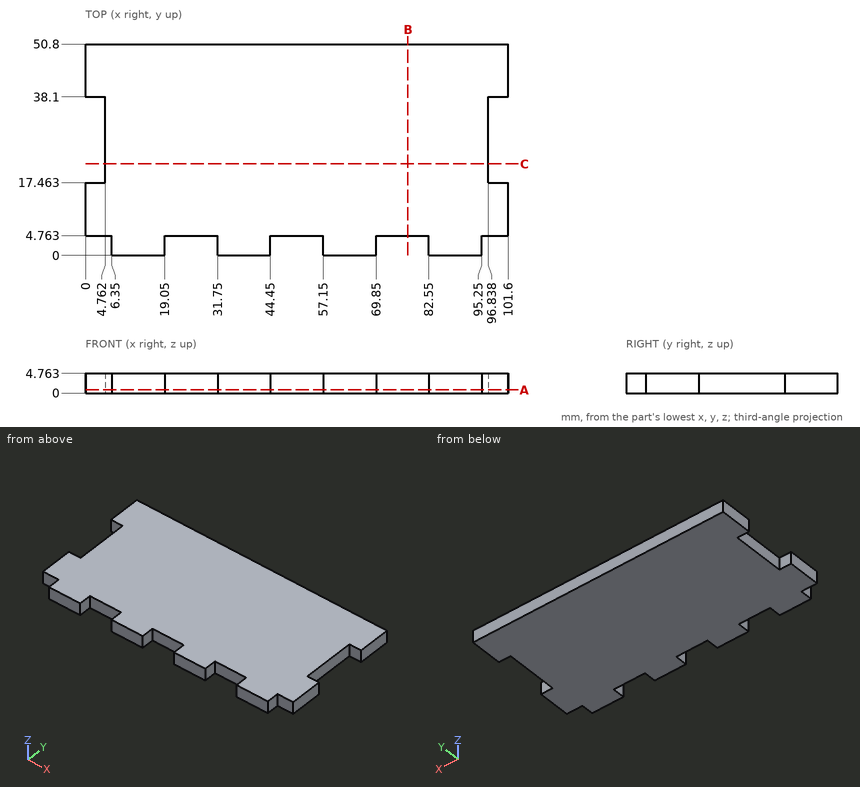
Design review of the part shown in the three views and the two pictorial views. Dimensions are in mm from the part's minimum x, y and z. Round coordinates to 2 decimals unless told otherwise and drop trailing zeros. Write each loop counter-clockwise with the first axis right and the second up, starting at its lowest first coordinate (ties: lowest second). Pieces come first, ordered by that corner, then holes. Notation, with made-up numbers: (28, 54) -> (75, 54) arc R26 cw to (75, 71) -> close; hole circle Ø2 at (19, -11). An arc over 180 degrees is marked (long way). Answer as a JSON object with one key per item and string values.
1. We need section C-C on y = 22. State the section outline as (x, z) points.
Results found:
{"outline": "(4.76, 0) -> (96.84, 0) -> (96.84, 4.76) -> (4.76, 4.76) -> close"}
2. We need section A-A on z = 0.8. State the section outline as (x, y) points, and give its area (3 significant figures).
Results found:
{"outline": "(0, 4.76) -> (6.35, 4.76) -> (6.35, 0) -> (19.05, 0) -> (19.05, 4.76) -> (31.75, 4.76) -> (31.75, 0) -> (44.45, 0) -> (44.45, 4.76) -> (57.15, 4.76) -> (57.15, 0) -> (69.85, 0) -> (69.85, 4.76) -> (82.55, 4.76) -> (82.55, 0) -> (95.25, 0) -> (95.25, 4.76) -> (101.6, 4.76) -> (101.6, 17.46) -> (96.84, 17.46) -> (96.84, 38.1) -> (101.6, 38.1) -> (101.6, 50.8) -> (0, 50.8) -> (0, 38.1) -> (4.76, 38.1) -> (4.76, 17.46) -> (0, 17.46) -> close", "area": "4,720 mm^2"}
3. Clearance check with flat-ended pins moving along their axes: pin 1 (1.4 mm diameter, centred on y = 1.5, z = 2.5, fed in from -X); pin 2 (6 mm diameter, centred on x = 42, y = 7.5, fed in from -Z); pin 3 (1.4 mm diameter, centred on x = 100.5, z = 3, fed in from -Y); pin 4 (1.4 mm diameter, centred on y = 23, z = 1.5, fed in from +X). State where each tip first meets the part, or that it passes through.
Results found:
{"pin 1": "stops at x = 6.35", "pin 2": "stops at z = 0", "pin 3": "stops at y = 4.76", "pin 4": "stops at x = 96.84"}
4. We need section B-B on x = 77.5. State the section outline as (y, z) points, and give its area (3 significant figures).
Results found:
{"outline": "(4.76, 0) -> (50.8, 0) -> (50.8, 4.76) -> (4.76, 4.76) -> close", "area": "219 mm^2"}
5. To check wall thickness, follow line 1 along X through (y, z) = (4, 4.4); line 2 along X through (y, z) = (27, 4.3); line 3 along Y through (x, z) = (80, 0.35). State the ranges of each line that lie inside material, in increasing order.
Results found:
{"line 1": "x = 6.35 to 19.05, 31.75 to 44.45, 57.15 to 69.85, 82.55 to 95.25", "line 2": "x = 4.76 to 96.84", "line 3": "y = 4.76 to 50.8"}
